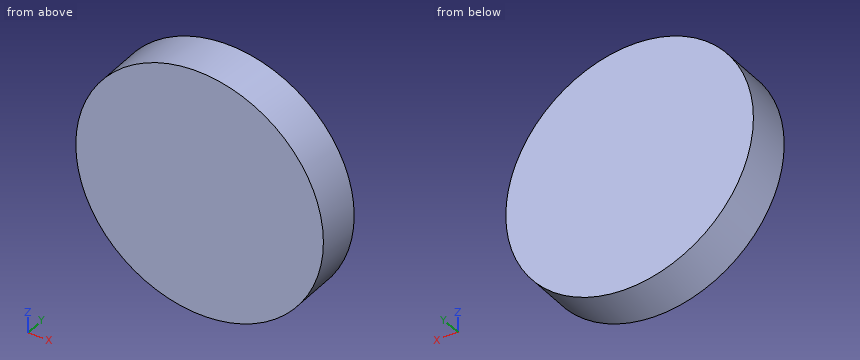
Autodesk Inventor part; units mm, degrees
ref_plane "YZ Plane" through (0, 0, 0) normal (1, 0, 0) x (0, 1, 0)
ref_plane "XZ Plane" through (0, 0, 0) normal (0, 1, 0) x (-1, 0, 0)
ref_plane "XY Plane" through (0, 0, 0) normal (0, 0, 1) x (1, 0, 0)
sketch "Szkic1" plane through (0, 0, 0) normal (0, 1, 0) x (-1, 0, 0)
  circle A0 centre (0, 0) radius 29.9
  arc A1 (42.6967, -16.4766) -> (42.6967, 16.4766) centre (36.8, 0) ccw
  arc A2 (-39.1229, 3.647) -> (-39.1229, -3.647) centre (-38.25, 0) ccw
  line L0 (42.6967, 16.4766) -> (10.075, 28.1515)
  line L1 (42.6967, -16.4766) -> (10.075, -28.1515)
  line L2 (-39.1229, 3.647) -> (-29.2918, 6)
  line L3 (-39.1229, -3.647) -> (-29.2918, -6)
  point P0 (54.3, 0)
  point P1 (29.9, 0)
  point P2 (-42, 0)
  dimension "d0" = 59.8
  dimension "d1" = 0
  dimension "d2" = 24.4
  dimension "d3" = 35
  dimension "d4" = 7.5
  dimension "d5" = 96.3
  dimension "d6" = 6
  dimension "d7" = 6
extrude "Wyciągnięcie proste2" add sketch "Szkic1" along normal blind 11 contours A0
properties part number "lidar"
Read the model definition and answer for the solid it produces. Units are mm, in the model's axes. Give positions to 0.01 mm unless a question says otherwise; leave off trailing zeros. Write each loop counter-clockwise with the first axis right and the second up, starting at its lowest first coordinate (ties: lowest second). Pieces come first, ordered by that corner, then holes. Notation, with made-up numbers: (-5.5, 72) -> (33.5, 72) arc R35 ccw to (33.5, 105) -> close; hole circle Ø11 at (-22.5, 15). An arc over 180 degrees is marked (long way). Answer as a JSON object with one key per item and string values. Group by question number.
1) Find section B-B (z = 25.5). Write down the section's boundary in (x, y), and give its area (3 significant figures).
2) Find section A-A (y = 1.25). Write down the section's boundary in (x, z).
3) Each of these flat-tipped pins is pushed along its axis until it touches: P1, Ø4, axis at y = 3, z = 4.5, coming from the +X side; P2, Ø4, axis at x = -8, z = 7.5, coming from the -Y side; P3, Ø1, axis at x = 21.5, y = 1.5, coming from the -Z side. Where does it stop, or does it pass through?
4) Find section C-C (x = -7). Write down the section's boundary in (y, z), and give its area (3 significant figures).
5) Consider L1, parallel to X at y = 5.75, z = 0.5; L2, parallel to Z at x = 13, y = 1; L3, parallel to Z at x = 3.5, y = 6.5. Determine where each line is inside the solid, lowest interval first. Write a range as from..to.
Values follow:
{
 "1": {"outline": "(-15.61, 0) -> (15.61, 0) -> (15.61, 11) -> (-15.61, 11) -> close", "area": "343 mm2"},
 "2": {"outline": "circle Ø59.8 at (0, 0)"},
 "3": {"P1": "stops at x = 29.8", "P2": "stops at y = 0", "P3": "stops at z = -21.28"},
 "4": {"outline": "(0, -29.07) -> (11, -29.07) -> (11, 29.07) -> (0, 29.07) -> close", "area": "640 mm2"},
 "5": {"L1": "x = -29.9..29.9", "L2": "z = -26.93..26.93", "L3": "z = -29.69..29.69"}
}
